Can you work these out from the model? Positions are in its coordinate system, mm. Coordinates: 2 decimals unless noted, no trailing zeros. Order: outer loops, then holes, each group sorted by start corner. A loop starts at its lowest first (then second) coordinate and runs counter-clockwise, first axis right, second up. Notation, with made-up numbers: (11.25, -22) - (50.25, -22) arc R17 cw to (50.25, 9) - close; hole circle Ø8 at (11.25, -9.5). An arc over 180 degrees is marked (long way). Return JSON: item names as keys, results as strings. Group by question number.
1) If I drill on line 1 along X through (y, z) = (-5.75, -11.5); line 2 along X through (y, z) = (-6, 11.75); line 3 along X through (y, z) = (-2.5, 4), over which ranges is the centre line in solid material (lowest first)?
2) Imagine slicing it at B-B (y = -2.5). Write out the boundary of the cut face in (x, z), and give its area (3 significant figures).
3) Imagine slicing it at A-A (z = 0). Write out the boundary of the cut face in (x, y), and give its area (3 significant figures).
4) Imagine slicing it at D-D (z = -6.25). Write out the boundary of the cut face in (x, y), and give its area (3 significant figures).
5) If we mould it in two halves opening along Z, with no side actions, what happens to faces 1 (the face through (-5, -4, -16.102)), 2 (the face through (33.485, -4, -1)), 3 (the face through (-39.46, -3.8, -13.56))? For each: pulls with the +Z half, pulls with the -Z half, needs draft (parallel to the pull), parting line crosses it, or undercut.
6) Imagine slicing it at C-C (x = -33). Write out the boundary of the cut face in (y, z).
```python
from build123d import *

# Parameters (mm, degrees)
F0_W     = 75
F0_H     = 30
F1_DEPTH = 7.5
F2_R     = 7.5
F3_DEPTH = 25
F4_R     = 7.5
F5_DEPTH = 25
F6_R     = 3
F7_DEPTH = 7.5


with BuildPart() as f1:
    # F0 (on Front) → F1 (new body)
    with BuildSketch(Plane.XZ):
        with Locations((-4.015371, -1.101968)):
            Rectangle(F0_W, F0_H)
    extrude(amount=F1_DEPTH)

    # F2 (on face) → F3 (cut)
    with BuildSketch(Plane(origin=(0, 0, 0), x_dir=(-1, 0, 0), z_dir=(0, 1, 0))):
        with Locations((-20.808353, 0)):
            Circle(F2_R)
    extrude(amount=-F3_DEPTH, mode=Mode.SUBTRACT)

    # F4 (on face) → F5 (cut)
    with BuildSketch(Plane.XZ.offset(7.5)):
        with Locations((-3.769332, 0)):
            Circle(F4_R)
        with Locations((-27.835064, 0)):
            Circle(F4_R)
    extrude(amount=-F5_DEPTH, mode=Mode.SUBTRACT)

    # F6 (on face) → F7 (cut, through all)
    with BuildSketch(Plane.XZ.offset(7.5)):
        with Locations((-36.896855, 9.086539)):
            Circle(F6_R)
        with Locations((-37.076353, -11.738191)):
            Circle(F6_R)
        with Locations((28.926538, 9.358378)):
            Circle(F6_R)
        with Locations((28.632505, -11.309632)):
            Circle(F6_R)
    extrude(amount=-F7_DEPTH, mode=Mode.SUBTRACT)


solid = f1.part
```
Calculated:
{
 "1": {"line 1": "-41.52 to -40.07, -34.09 to 25.64, 31.63 to 33.48", "line 2": "-41.52 to -38.28, -35.52 to 27.12, 30.74 to 33.48", "line 3": "-41.52 to -34.18, -21.49 to -10.11, 2.57 to 14.46, 27.15 to 33.48"},
 "2": {"outline": "(-41.52, -16.1) - (33.48, -16.1) - (33.48, 13.9) - (-41.52, 13.9) - close; hole circle Ø6 at (-37.08, -11.74); hole circle Ø6 at (-36.9, 9.09); hole circle Ø15 at (-27.84, 0); hole circle Ø15 at (-3.77, 0); hole circle Ø15 at (20.81, 0); hole circle Ø6 at (28.63, -11.31); hole circle Ø6 at (28.93, 9.36)", "area": "1,610 mm2"},
 "3": {"outline": "(-41.52, -7.5) - (-35.34, -7.5) - (-35.34, 0) - (-41.52, 0) - close; (-20.34, -7.5) - (-11.27, -7.5) - (-11.27, 0) - (-20.34, 0) - close; (3.73, -7.5) - (13.31, -7.5) - (13.31, 0) - (3.73, 0) - close; (28.31, -7.5) - (33.48, -7.5) - (33.48, 0) - (28.31, 0) - close", "area": "225 mm2"},
 "4": {"outline": "(-41.52, -7.5) - (-31.98, -7.5) - (-31.98, 0) - (-41.52, 0) - close; (-23.69, -7.5) - (-7.92, -7.5) - (-7.92, 0) - (-23.69, 0) - close; (0.38, -7.5) - (16.66, -7.5) - (16.66, 0) - (0.38, 0) - close; (24.95, -7.5) - (33.48, -7.5) - (33.48, 0) - (24.95, 0) - close", "area": "376 mm2"},
 "5": {"face 1": "pulls with the -Z half", "face 2": "needs draft", "face 3": "undercut"},
 "6": {"outline": "(-7.5, -16.1) - (0, -16.1) - (0, -5.44) - (-7.5, -5.44) - close; (-7.5, 5.44) - (0, 5.44) - (0, 13.9) - (-7.5, 13.9) - close"}
}
